```python
from build123d import *

# Parameters (mm, degrees)
F0_R     = 225
F0_R_2   = 127.5080178576
F1_DEPTH = 125
F0_R_3   = 21
F2_DEPTH = 2.5
F3_R     = 20


# Not quite as in the source:
# - a fillet or chamfer that OpenCascade refuses, or shapes differently, is made with other operations: its cross-section is extruded or revolved along the edge and cut away or added


with BuildPart() as f1:
    # F0 (on Right) → F1 (new body, symmetric)
    with BuildSketch(Plane.YZ):
        Circle(F0_R)
        Circle(F0_R_2, mode=Mode.SUBTRACT)
    extrude(amount=F1_DEPTH, both=True)

    # F0 (on Right) → F2 (join, symmetric)
    with BuildSketch(Plane.YZ):
        Circle(F0_R_2)
        Circle(F0_R_3, mode=Mode.SUBTRACT)
    extrude(amount=F2_DEPTH, both=True)

    # F3
    f3_edges = [f1.edges().sort_by_distance(p)[0] for p in [
        (125, -225, 0),
    ]]
    fillet(f3_edges, radius=F3_R)

    # F4: chamfer of 20 on 5 edges, made by hand

    # F4_s1 → F4_t2 (revolve)
    with BuildSketch(Plane.XY):
        Polygon((-22.5, 127.5080178576), (-2.5, 107.5080178576), (-2.5, 127.5080178576), align=None)
    revolve(axis=Axis((-2.5, 0, 0), (1, 0, 0)))

    # F4_s3 → F4_t4 (revolve)
    with BuildSketch(Plane.XY):
        Polygon((22.5, 127.5080178576), (2.5, 107.5080178576), (2.5, 127.5080178576), align=None)
    revolve(axis=Axis((2.5, 0, 0), (1, 0, 0)))

    # F4_s5 → F4_t6 (revolve, cut)
    with BuildSketch(Plane.XY):
        Polygon((-125, 147.5080178576), (-105, 127.5080178576), (-125, 127.5080178576), align=None)
    revolve(axis=Axis((-125, 0, 0), (1, 0, 0)), mode=Mode.SUBTRACT)

    # F4_s7 → F4_t8 (revolve, cut)
    with BuildSketch(Plane.XY):
        Polygon((125, 147.5080178576), (105, 127.5080178576), (125, 127.5080178576), align=None)
    revolve(axis=Axis((125, 0, 0), (1, 0, 0)), mode=Mode.SUBTRACT)

    # F4_s9 → F4_t10 (revolve, cut)
    with BuildSketch(Plane.XY):
        Polygon((2.5, 41), (-17.5, 21), (2.5, 21), align=None)
    revolve(axis=Axis((2.5, 0, 0), (1, 0, 0)), mode=Mode.SUBTRACT)


solid = f1.part
```
Work out the finished part from the listing and answer in its coordinate system (mm). A direction names the side the tool comes from. Give positions to 0.01 mm unless a question says otherwise; leave off trailing zeros. Loops run counter-clockwise (first coordinate to the right, second up) from the corner with the lowest first, then second, coordinate; pieces in that order, holes last. Notation, with made-up numbers: (78, 37.25) -> (127, 37.25) arc R17 cw to (127, 51.25) -> close; hole circle Ø9 at (5, -10.75). An arc over 180 degrees is marked (long way). Write item = value, one per line. Start each with the question number.
(1) Which of the six approach directions +Z, -Z, +X, -X, +Y, -Y give full straight-line access (tool end or side, diameter ignored) to faces 5 (the flat face through (-2.5, 46, 2)), 6 (the cylindrical face through (63.17, 121.62, 38.3)), 7 (the flat face through (-125, 47, -147))?
(2) Given pin 1 Ø5 at (x, z) = (28.5, -103) entering from +Y; pin 2 Ø10 at (y, z) = (-74, 0.5) entering from -X; pin 3 Ø12 at (y, z) = (-116.5, 70.5) entering from +X, each flat-ended and moving along its own axis, determine where each tip first touches the part or whether it passes through.
(3) Find the intervals of material crossed by probe 1 along Z at (x, y) = (68, 0); probe 2 along X at (y, z) = (102, -22.5); probe 3 along Y at (x, z) = (-67, -13), in increasing order. Write a range as from..to.
(4) Find section C-C on x = -89. Give the vertices of the cut face in (y, z), and give its area (3 significant figures).
(5) Find section D-D on x = -8.5. Give the vertices of the cut face in (y, z).
(6) The mould has two halves that part along Y. Classify faces 1 (the flat face through (125, -140, 48)), 2 (the conical face through (-2.26, -7.86, -35.38)), 3 (the cylindrical face through (-8.39, -224.782, 9.893)), 4 (the conical face through (105.971, 122.546, 38.592)): +Y half, -Y half, draft (parallel to the pull), parting line (faces both ways), or undercut.
(7) Find section A-A on y = 0. Give the vertices of the cut face in (x, z), and give its area (3 significant figures).
From the geometry:
q1.face_5 = -X
q1.face_6 = +X
q1.face_7 = +Z, -Z, -X, +Y, -Y
q2.pin_1 = 201.31
q2.pin_2 = -2.5
q2.pin_3 = 119.66
q3.probe_1 = -225..-127.51, 127.51..225
q3.probe_2 = -2.5..2.5
q3.probe_3 = -224.62..-126.84, 126.84..224.62
q4.outline = circle Ø450 at (0, 0); hole circle Ø255.02 at (0, 0)
q4.area = 108,000 mm^2
q5.outline = circle Ø450 at (0, 0); hole circle Ø227.02 at (0, 0)
q6.face_1 = draft
q6.face_2 = undercut
q6.face_3 = parting line
q6.face_4 = undercut
q7.outline = (-125, -225) -> (105, -225) arc R20 ccw to (125, -205) -> (125, -147.51) -> (105, -127.51) -> (22.5, -127.51) -> (2.5, -107.51) -> (2.5, -41) -> (-2.5, -36) -> (-2.5, -107.51) -> (-22.5, -127.51) -> (-105, -127.51) -> (-125, -147.51) -> close; (-125, 147.51) -> (-105, 127.51) -> (-22.5, 127.51) -> (-2.5, 107.51) -> (-2.5, 36) -> (2.5, 41) -> (2.5, 107.51) -> (22.5, 127.51) -> (105, 127.51) -> (125, 147.51) -> (125, 205) arc R20 ccw to (105, 225) -> (-125, 225) -> close
q7.area = 49,500 mm^2
